The model under review builds one solid part; all positions refer to its coordinate system, in mm. A direction names the side the tool comes from. Coordinates: 2 decimals unless noted, no trailing zeros. Order: outer loops, then holes, each group sorted by start corner. A loop starts at its lowest first (then second) coordinate and runs counter-clockwise, first axis right, second up. Notation, with made-up numbers: (33.25, 60.5) -> (90.25, 60.5) arc R7 cw to (90.25, 68.5) -> close; hole circle Ø4 at (-5.75, -14). An arc over 180 degrees is marked (long way). Use one line per item in the form item = value. Start each with the question number.
(1) Take a section at C-C (y = 6.5). State the section outline as (x, z) points.
(2) For faces 1 (the flat face through (30.375, -16, 10)), 2 (the flat face through (10, 7, 11.893)), 3 (the flat face through (13.309, 7, 10)), 4 (the flat face through (5.928, 7, 10)), 5 (the flat face through (10, 7, 7.771)), list the 3-axis set-ups (+Z, -Z, +X, -X, +Y, -Y) from which the entire face can be reached by the end or side of a thin tool; tool diameter is ignored.
(3) Take a section at B-B (x = 23). State the section outline as (y, z) points, then the cut area to 3 significant figures.
(4) Take a section at A-A (z = 9.25). State the section outline as (x, y) points (3 decimals).
(5) Wall thickness on line 1 along Y through (x, z) = (-1.5, 11); line 2 along Z through (x, y) = (7, 11); line 3 along Z through (x, y) = (-3, -24): over which ranges is each line inside the solid? List them lowest first.
(6) Insertion check: pin 1 Ø10 at (x, z) = (24, 4.5) entering from +Y; pin 2 Ø8 at (x, y) = (9, 8) entering from -Z; pin 3 Ø6 at (x, z) = (12, 7) entering from +Y (3 decimals); pin 4 Ø3.5 at (x, y) = (11, 7.5) entering from +Z. Each pin has a flat end and moves straight along its axis. Give the tip position at first contact, or say it passes through.
(7) Take a section at D-D (x = 12). State the section outline as (y, z) points (3 decimals), then the cut area to 3 significant figures.
```python
from build123d import *

# Parameters (mm, degrees)
F0_W     = 44.029299
F0_H     = 20.568207
F1_DEPTH = 31.881519
F2_R     = 8.141147
F3_W     = 7.381364
F3_H     = 4.12172
F4_DEPTH = 13.804998


with BuildPart() as f1:
    # F0 (on Front) → F1 (new body)
    with BuildSketch(Plane.XZ):
        with Locations((8.360238, 10.284103)):
            Rectangle(F0_W, F0_H)
    extrude(amount=F1_DEPTH)

    # F2
    f2_edges = [f1.edges().sort_by_distance(p)[0] for p in [
        (8.360239, -31.881519, 20.568207),
    ]]
    fillet(f2_edges, radius=F2_R)

    # F3 (on face) → F4 (join)
    with BuildSketch(Plane(origin=(0, 0, 0), x_dir=(-1, 0, 0), z_dir=(0, 1, 0))):
        with Locations((-9.618722, 9.832263)):
            Rectangle(F3_W, F3_H)
    extrude(amount=F4_DEPTH)


solid = f1.part
```
Findings:
q1.outline = (5.93, 7.77) -> (13.31, 7.77) -> (13.31, 11.89) -> (5.93, 11.89) -> close
q2.face_1 = +Z, -Z, +X, +Y, -Y
q2.face_2 = +Z, +X, -X, +Y
q2.face_3 = +Z, -Z, +X, +Y
q2.face_4 = +Z, -Z, -X, +Y
q2.face_5 = -Z, +X, -X, +Y
q3.outline = (-31.88, 0) -> (0, 0) -> (0, 20.57) -> (-23.74, 20.57) arc R8.14 ccw to (-31.88, 12.43) -> close
q3.area = 642 mm²
q4.outline = (-13.654, -31.882) -> (30.375, -31.882) -> (30.375, 0) -> (13.309, 0) -> (13.309, 13.805) -> (5.928, 13.805) -> (5.928, 0) -> (-13.654, 0) -> close
q5.line_1 = -31.88 to 0
q5.line_2 = 7.77 to 11.89
q5.line_3 = 0 to 20.56
q6.pin_1 = 0
q6.pin_2 = 7.77
q6.pin_3 = 13.805
q6.pin_4 = 11.89
q7.outline = (-31.882, 0) -> (0, 0) -> (0, 7.771) -> (13.805, 7.771) -> (13.805, 11.893) -> (0, 11.893) -> (0, 20.568) -> (-23.74, 20.568) arc R8.141 ccw to (-31.882, 12.427) -> close
q7.area = 698 mm²
